The model under review builds one solid part; all positions refer to its coordinate system, in mm. Coordinates: 2 decimals unless noted, no trailing zeros.
from build123d import *

# Parameters (mm, degrees)
SKETCH_1_W          = 400
SKETCH_1_H          = 60
SKETCH_1_R          = 1.6
SKETCH_1_W_2        = 21
SKETCH_1_H_2        = 21
SKETCH_1_W_3        = 240
SKETCH_1_H_3        = 75
SKETCH_1_R_2        = 20
EXTRUDE_1468_DEPTH  = 3
SKETCH_2_R          = 2.05
SKETCH_2_R_2        = 2.1
CUT_EXTRUDE_1_DEPTH = 250.229009796
FILLET_1_R          = 5
SKETCH1_R           = 2.1
CUT_EXTRUDE4_DEPTH  = 250.229009796
CUT_EXTRUDE_2_DEPTH = 10


with BuildPart() as part:
    # 草图1 → Extrude 1468 (new body)
    # profile 1 of 2: a face of its own
    with BuildSketch(Plane(origin=(0, 0, 0), x_dir=(1, 0, 0), z_dir=(0, 1, 0))):
        with Locations((32.825924772, 16.128249268)):
            Rectangle(SKETCH_1_W, SKETCH_1_H)
        with Locations(Location((-14.674075228, 36.128249268, 0), (0, 0, 270))):
            Circle(SKETCH_1_R, mode=Mode.SUBTRACT)
        with Locations(Location((-14.674075228, 11.128249268, 0), (0, 0, 270))):
            Circle(SKETCH_1_R, mode=Mode.SUBTRACT)
        with Locations(Location((80.325924772, 11.128249268, 0), (0, 0, 270))):
            Circle(SKETCH_1_R, mode=Mode.SUBTRACT)
        with Locations(Location((80.325924772, 36.128249268, 0), (0, 0, 270))):
            Circle(SKETCH_1_R, mode=Mode.SUBTRACT)
        with Locations((32.825924772, 10.628249268)):
            Rectangle(SKETCH_1_W_2, SKETCH_1_H_2, mode=Mode.SUBTRACT)
    # profile 2 of 2: a face of its own
    with BuildSketch(Plane(origin=(0, 0, 0), x_dir=(1, 0, 0), z_dir=(0, 1, 0))):
        with Locations((32.825924772, -51.371750732)):
            Rectangle(SKETCH_1_W_3, SKETCH_1_H_3)
        with Locations(Location((7.825924772, -29.871750732, 0), (0, 0, 270))):
            Circle(SKETCH_1_R, mode=Mode.SUBTRACT)
        with Locations(Location((7.825924772, -79.871750732, 0), (0, 0, 270))):
            Circle(SKETCH_1_R, mode=Mode.SUBTRACT)
        with Locations(Location((57.825924772, -79.871750732, 0), (0, 0, 270))):
            Circle(SKETCH_1_R, mode=Mode.SUBTRACT)
        with Locations(Location((57.825924772, -29.871750732, 0), (0, 0, 270))):
            Circle(SKETCH_1_R, mode=Mode.SUBTRACT)
        with Locations(Location((32.825924772, -54.871750732, 0), (0, 0, 270))):
            Circle(SKETCH_1_R_2, mode=Mode.SUBTRACT)
    extrude(amount=EXTRUDE_1468_DEPTH)

    # 草图2 → 切除-拉伸1 (cut, through all)
    with BuildSketch(Plane(origin=(0, 3, 0), x_dir=(1, 0, 0), z_dir=(0, 1, 0))):
        with Locations(Location((-149.174075228, 29.628249268, 0), (0, 0, 270))):
            Circle(SKETCH_2_R)
        with Locations(Location((-149.174075228, 2.628249268, 0), (0, 0, 270))):
            Circle(SKETCH_2_R)
        with Locations(Location((-121.674075228, 29.628249268, 0), (0, 0, 270))):
            Circle(SKETCH_2_R)
        with Locations(Location((-121.674075228, 2.628249268, 0), (0, 0, 90))):
            Circle(SKETCH_2_R)
        with Locations(Location((-51.674075228, 41.128249268, 0), (0, 0, 270))):
            Circle(SKETCH_2_R_2)
        with Locations(Location((-86.674075228, 41.128249268, 0), (0, 0, 270))):
            Circle(SKETCH_2_R_2)
        with Locations(Location((-51.674075228, -8.871750732, 0), (0, 0, 90))):
            Circle(SKETCH_2_R_2)
        with Locations(Location((-86.674075228, -8.871750732, 0), (0, 0, 90))):
            Circle(SKETCH_2_R_2)
        with Locations(Location((-135.424075228, 41.128249268, 0), (0, 0, 270))):
            Circle(SKETCH_2_R_2)
        with Locations(Location((-135.424075228, -8.871750732, 0), (0, 0, 90))):
            Circle(SKETCH_2_R_2)
        with Locations(Location((201.075924772, -8.871750732, 0), (0, 0, 270))):
            Circle(SKETCH_2_R_2)
        with Locations(Location((201.075924772, 41.128249268, 0), (0, 0, 90))):
            Circle(SKETCH_2_R_2)
        with Locations(Location((152.325924772, -8.871750732, 0), (0, 0, 270))):
            Circle(SKETCH_2_R_2)
        with Locations(Location((117.325924772, -8.871750732, 0), (0, 0, 270))):
            Circle(SKETCH_2_R_2)
        with Locations(Location((152.325924772, 41.128249268, 0), (0, 0, 90))):
            Circle(SKETCH_2_R_2)
        with Locations(Location((117.325924772, 41.128249268, 0), (0, 0, 90))):
            Circle(SKETCH_2_R_2)
        with Locations(Location((187.325924772, 2.628249268, 0), (0, 0, 270))):
            Circle(SKETCH_2_R)
        with Locations(Location((187.325924772, 29.628249268, 0), (0, 0, 90))):
            Circle(SKETCH_2_R)
        with Locations(Location((214.825924772, 2.628249268, 0), (0, 0, 90))):
            Circle(SKETCH_2_R)
        with Locations(Location((214.825924772, 29.628249268, 0), (0, 0, 90))):
            Circle(SKETCH_2_R)
    extrude(amount=-CUT_EXTRUDE_1_DEPTH, mode=Mode.SUBTRACT)

    # 圆角1
    fillet_1_edges = [part.edges().sort_by_distance(p)[0] for p in [
        (-167.174075228, 1.5, 13.871750732),
        (-167.174075228, 1.5, -46.128249268),
        (232.825924772, 1.5, -46.128249268),
        (232.825924772, 1.5, 13.871750732),
        (152.825924772, 1.5, 13.871750732),
        (152.825924772, 1.5, 88.871750732),
        (-87.174075228, 1.5, 88.871750732),
        (-87.174075228, 1.5, 13.871750732),
    ]]
    fillet(fillet_1_edges, radius=FILLET_1_R)

    # Sketch1 → Cut-Extrude4 (cut, through all)
    with BuildSketch(Plane(origin=(0, 0, 0), x_dir=(1, 0, 0), z_dir=(0, 1, 0))):
        with Locations(Location((-72.174075228, -33.871750732, 0), (0, 0, 270))):
            Circle(SKETCH1_R)
        with Locations(Location((-72.174075228, -68.871750732, 0), (0, 0, 270))):
            Circle(SKETCH1_R)
        with Locations(Location((137.825924772, -68.871750732, 0), (0, 0, 90))):
            Circle(SKETCH1_R)
        with Locations(Location((137.825924772, -33.871750732, 0), (0, 0, 90))):
            Circle(SKETCH1_R)
        with BuildLine():
            Line((-42.174075228, -68.871750732), (-42.174075228, -33.871750732))
            ThreePointArc((-42.174075228, -33.871750732), (-32.174075228, -23.871750732), (-22.174075228, -33.871750732))
            Line((-22.174075228, -33.871750732), (-22.174075228, -68.871750732))
            ThreePointArc((-22.174075228, -68.871750732), (-32.174075228, -78.871750732), (-42.174075228, -68.871750732))
        make_face()
        with BuildLine():
            Line((107.825924772, -68.871750732), (107.825924772, -33.871750732))
            ThreePointArc((107.825924772, -33.871750732), (97.825924772, -23.871750732), (87.825924772, -33.871750732))
            Line((87.825924772, -33.871750732), (87.825924772, -68.871750732))
            ThreePointArc((87.825924772, -68.871750732), (97.825924772, -78.871750732), (107.825924772, -68.871750732))
        make_face()
    extrude(amount=CUT_EXTRUDE4_DEPTH, mode=Mode.SUBTRACT)

    # 草图3 → 切除-拉伸2 (cut)
    with BuildSketch(Plane(origin=(0, 3, 0), x_dir=(1, 0, 0), z_dir=(0, 1, 0))):
        with BuildLine():
            ThreePointArc((157.825924772, -13.871750732), (154.290390866, -15.336216826), (152.825924772, -18.871750732))
            Line((152.825924772, -18.871750732), (152.825924772, -83.871750732))
            ThreePointArc((152.825924772, -83.871750732), (151.361458678, -87.407284637), (147.825924772, -88.871750732))
            Line((147.825924772, -88.871750732), (-82.174075228, -88.871750732))
            ThreePointArc((-82.174075228, -88.871750732), (-85.709609134, -87.407284637), (-87.174075228, -83.871750732))
            Line((-87.174075228, -83.871750732), (-87.174075228, -18.871750732))
            ThreePointArc((-87.174075228, -18.871750732), (-88.638541322, -15.336216826), (-92.174075228, -13.871750732))
            Line((-92.174075228, -13.871750732), (157.825924772, -13.871750732))
        make_face()
    extrude(amount=-CUT_EXTRUDE_2_DEPTH, mode=Mode.SUBTRACT)


solid = part.part
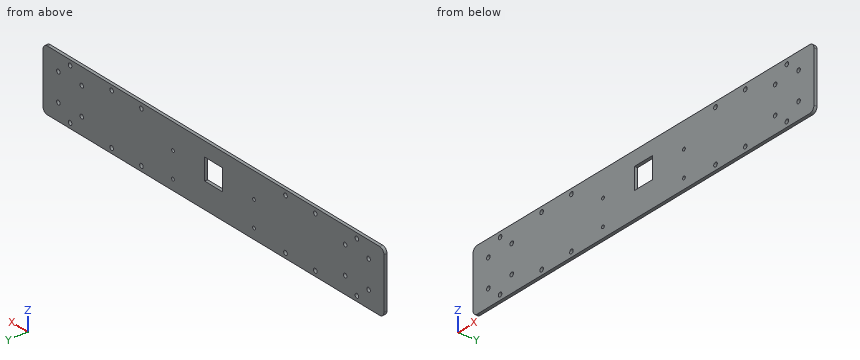
(1) Wall thickness on line 1 (X direction, y = 0.95, z = -11); line 2 (Z direction, x = 187, y = 1.8); line 3 (Z direction, x = 24.5, y = 1.1): over which ranges is each line inside the solid? List them lowest first.
(2) Consider section A-A (y = 0.9). Give the number of separate pieces and of enclosed holes in the cut face, then the cut area to 3 significant figures.
(3) Insertion check: pin 1 Ø3.5 at (x, z) = (-121.67, -2.63) entering from -Y; pin 2 Ø3.5 at (x, z) = (80.33, -36.13) entering from +Y. Each pin has a flat end and moves straight along its axis. Give the tip position at first contact, or say it passes through.
Findings:
1. line 1: x = -167.17 to -16.27, -13.08 to 22.33, 43.33 to 78.73, 81.92 to 232.83
1. line 2: z = -46.13 to -31.65, -27.6 to -4.65, -0.6 to 13.87
1. line 3: z = -46.13 to -21.13, -0.13 to 13.87
2. separate pieces: 1
2. enclosed holes: 25
2. area: 23,200 mm2
3. pin 1: passes through
3. pin 2: stops at y = 3
